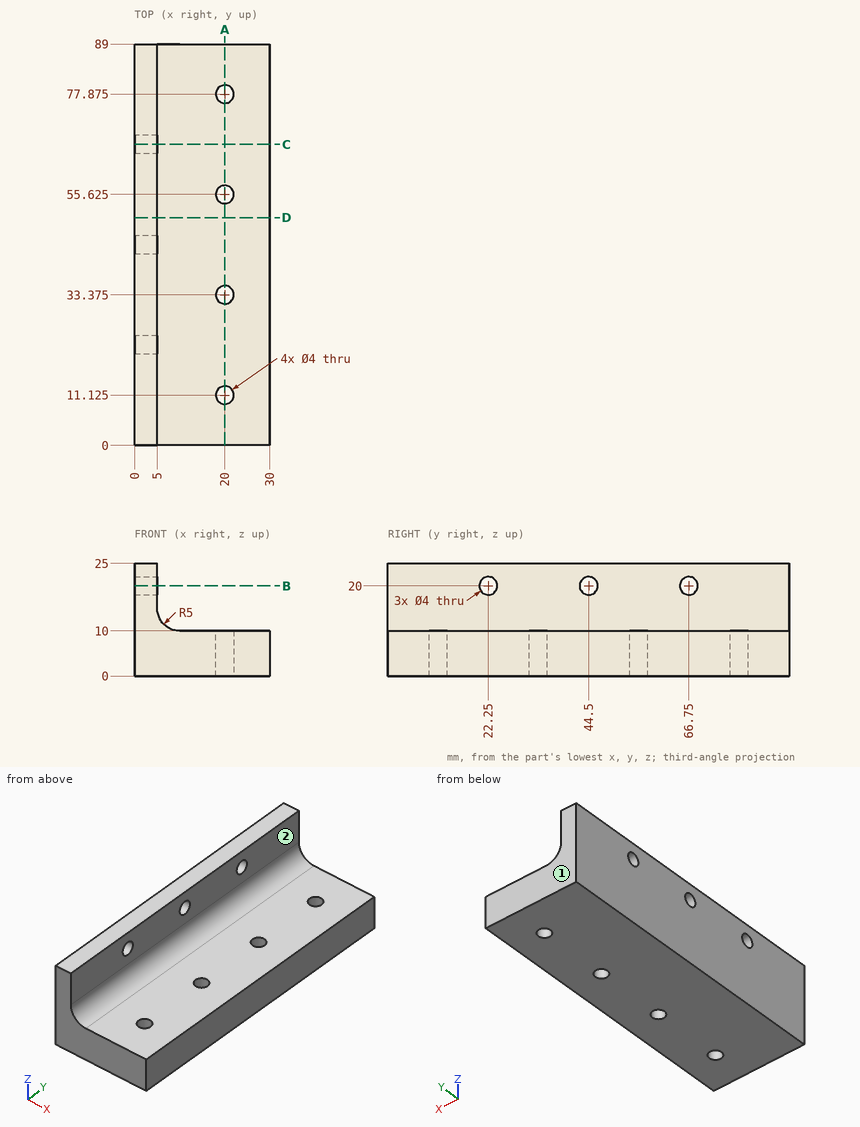
Source: three-view drawing plus pictorial views. Frame: mm from the lowest corner of the part. A direction names the side the tool comes from. Coordinates: 2 decimals unless noted, no trailing zeros. Loops run counter-clockwise (first coordinate to the right, second up) from the corner with the lowest first, then second, coordinate; pieces in that order, holes last. Notation, with made-up numbers: (50, 7) - (94, 7) arc R31 ccw to (94, 31) - close; hole circle Ø7 at (-17, 24). An arc over 180 degrees is marked (long way). Answer in a Markdown table with one row per item. Add a question column.
Item 1: Section query B-B on z = 20. Return the cut outline in (x, y), then the cut area to 3 significant figures.
Item 2: Section query A-A on x = 20. Return the cut outline in (y, z) (3 decimals), then the cut area to 3 significant figures.
Item 3: Access query for the marked faces 1 and 2. Directions: +Z, -Z, +X, -X, +Y, -Y. A direction counts if a zero-diameter tool reaches every point of the face in a straight line with its end or side. Return the directions, or none.
Item 4: Section query D-D on y = 50.5. Return the cut outline in (x, z).
Item 5: Contact query for flat-ended pins moving along their axis: P1, Ø4.5, axis at x = 20, y = 77.875, coming from the -Z side; P2, Ø6, axis at x = 24.5, y = 22.5, coming from the +Z side; P3, Ø8, axis at y = 22.5, z = 19, coming from the +X side; P4, Ø4, axis at x = 10.5, y = 67, coming from the +Z side. Output: stop coordinate, or through.
Item 6: Section query C-C on y = 66.75. Return the cut outline in (x, z).
Item 7: Line query: line 1 along Y through (x, z) = (20, 5.25) (3 decimals); line 2 along Z through (x, y) = (17.25, 76); line 3 along Z through (x, y) = (1.5, 44.5). Output: solid intervals per line, ascending. Write a range as [from, to].
Recorded:
| question | item | result |
|---|---|---|
| 1 | outline | (0, 0) - (5, 0) - (5, 20.25) - (0, 20.25) - close; (0, 24.25) - (5, 24.25) - (5, 42.5) - (0, 42.5) - close; (0, 46.5) - (5, 46.5) - (5, 64.75) - (0, 64.75) - close; (0, 68.75) - (5, 68.75) - (5, 89) - (0, 89) - close |
| 1 | area | 385 mm^2 |
| 2 | outline | (0, 0) - (9.125, 0) - (9.125, 10) - (0, 10) - close; (13.125, 0) - (31.375, 0) - (31.375, 10) - (13.125, 10) - close; (35.375, 0) - (53.625, 0) - (53.625, 10) - (35.375, 10) - close; (57.625, 0) - (75.875, 0) - (75.875, 10) - (57.625, 10) - close; (79.875, 0) - (89, 0) - (89, 10) - (79.875, 10) - close |
| 2 | area | 730 mm^2 |
| 3 | face 1 | +Z, -Z, +X, -X, +Y |
| 3 | face 2 | +Z, +X, +Y, -Y |
| 4 | outline | (0, 0) - (30, 0) - (30, 10) - (10, 10) arc R5 cw to (5, 15) - (5, 25) - (0, 25) - close |
| 5 | P1 | z = 0 |
| 5 | P2 | z = 10 |
| 5 | P3 | x = 5 |
| 5 | P4 | z = 10.23 |
| 6 | outline | (0, 0) - (30, 0) - (30, 10) - (10, 10) arc R5 cw to (5, 15) - (5, 18) - (0, 18) - close; (0, 22) - (5, 22) - (5, 25) - (0, 25) - close |
| 7 | line 1 | [0, 9.125], [13.125, 31.375], [35.375, 53.625], [57.625, 75.875], [79.875, 89] |
| 7 | line 2 | [0, 10] |
| 7 | line 3 | [0, 18], [22, 25] |
